Geometry check sheet. Reference: the model listing, model coordinates, mm. Face numbers are marked on the shaded views. Give positions to 0.01 mm unless a question says otherwise; leave off trailing zeros. Loops run counter-clockwise (first coordinate to the right, second up) from the corner with the lowest first, then second, coordinate; pieces in that order, holes last. Notation, with made-up numbers: (14.25, 32) - (21.25, 32) arc R20 ccw to (21.25, 48) - close; hole circle Ø6 at (22, 9.25). An arc over 180 degrees is marked (long way). Use a Markdown table: item, result. Add a question column.
1. Cross-section at B-B on y = -20. Enter the section's corners in (x, z), and give its area (3 significant figures).
2. Cross-section at C-C on x = 16.5. Enter the section's corners in (y, z).
3. Draft check along X on the marked faces 1, 2 and 3. Enter one of: pulls with the +X half, pulls with the -X half, needs draft (parallel to the pull), parting line crosses it, or undercut.
4. Material ranges on L1, parallel to Y at x = 0, z = 53; L2, parallel to Z at x = -19, y = 8; L3, parallel to Y at x = -5, z = 5, recorded low to high.
5. Cross-section at A-A on z = 35. Enter the section's corners in (x, y), and give its area (3 significant figures).
6. Depth check by flat-ended pin: P1, Ø1.5, axis at x = -2.5, y = 15, coming from the -Z side; P2, Ø5, axis at x = -5.5, z = 68.5, coming from the +Y side; P3, Ø6, axis at y = -3, z = 65.5, coming from the -X side. Enter the tip coordinate at first touch or a pass-through.
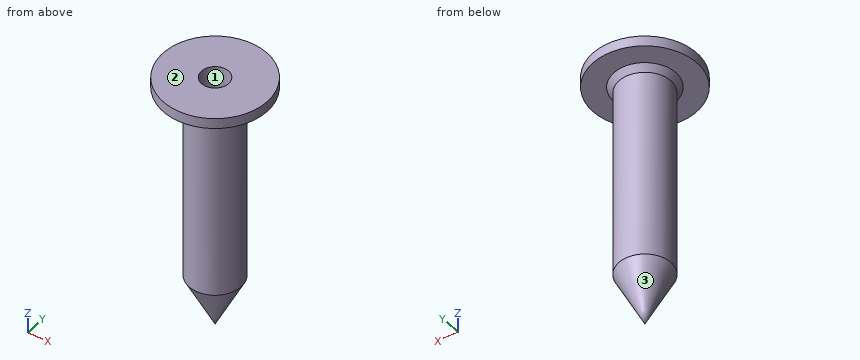
from build123d import *

# Parameters (mm, degrees)
F0_R     = 12.5
F0_R_2   = 6.5
F1_DEPTH = 100


with BuildPart() as f1:
    # F0 (on Top) → F1 (new body)
    with BuildSketch(Plane.XY):
        Circle(F0_R)
        Circle(F0_R_2, mode=Mode.SUBTRACT)
    extrude(amount=F1_DEPTH)

    # F2 (on Front) → F3 (revolve)
    with BuildSketch(Plane.XZ):
        Polygon((12.5, 0), (0, 0), (0, -25), align=None)
    revolve(axis=Axis((0, 0, -12.5), (0, 0, -1)))

    # F4 (on Front) → F5 (revolve)
    with BuildSketch(Plane.XZ):
        Polygon((14.8862302303, 95), (10, 95), (10, 89.0116691589), align=None)
        Polygon((25, 100), (10, 100), (10, 95), (14.8862302303, 95), (25, 95), align=None)
    revolve(axis=Axis((0, 0, 50), (0, 0, 1)))


solid = f1.part
Values found:
| question | item | result |
|---|---|---|
| 1 | outline | (-15, 95) - (15, 95) - (15, 100) - (-15, 100) - close |
| 1 | area | 150 mm2 |
| 2 | outline | (-18.78, 95) - (18.78, 95) - (18.78, 100) - (-18.78, 100) - close |
| 3 | face 1 | undercut |
| 3 | face 2 | needs draft |
| 3 | face 3 | parting line crosses it |
| 4 | L1 | y = -12.5 to -6.5, 6.5 to 12.5 |
| 4 | L2 | z = 95 to 100 |
| 4 | L3 | y = -11.46 to -4.15, 4.15 to 11.46 |
| 5 | outline | circle Ø25 at (0, 0); hole circle Ø13 at (0, 0) |
| 5 | area | 358 mm2 |
| 6 | P1 | stops at z = 94.47 |
| 6 | P2 | stops at y = 12.13 |
| 6 | P3 | stops at x = -12.5 |
